Autodesk Inventor part; units mm, degrees
ref_plane "YZ Plane" through (0, 0, 0) normal (1, 0, 0) x (0, 1, 0)
ref_plane "XZ Plane" through (0, 0, 0) normal (0, 1, 0) x (-1, 0, 0)
ref_plane "XY Plane" through (0, 0, 0) normal (0, 0, 1) x (1, 0, 0)
sketch "スケッチ1" plane through (0, 0, 0) normal (0, 1, 0) x (-1, 0, 0)
  circle A0 centre (0, 0) radius 1.15
  circle A1 centre (0, 0) radius 1
  circle A2 centre (0, 0) radius 1.5
  circle A3 centre (0, 0) radius 2
  line L0 (1.5, 0) -> (1, 0)
  line L1 (1, 0) -> (1, 2)
  line L2 (1, 2) -> (1.5, 2)
  line L3 (1.5, 2) -> (1.5, 0)
  line L4 (0, 0) -> (5, 0)
  line L5 (5, 0) -> (5, -5)
  line L6 (5, -5) -> (0, -5)
  line L7 (0, -5) -> (0, 0)
  line L8 (5, -5) -> (0, -5)
  line L9 (0, -5) -> (0, 5)
  line L10 (0, 5) -> (5, 5)
  line L11 (5, 5) -> (5, -5)
  line L12 (0, 0) -> (-2, 0)
  line L13 (-2, 0) -> (-2, -5)
  line L14 (-2, -5) -> (0, -5)
  line L15 (0, -5) -> (0, 0)
  line L16 (-2, -5) -> (1.5, -5)
  line L17 (1.5, -5) -> (1.5, -1.5)
  line L18 (1.5, -1.5) -> (-2, -1.5)
  line L19 (-2, -1.5) -> (-2, -5)
  line L20 (1.5, 2) -> (-2, 2)
  line L21 (-2, 2) -> (-2, 5)
  line L22 (-2, 5) -> (1.5, 5)
  line L23 (1.5, 5) -> (1.5, 2)
  line L24 (-2, 2) -> (1.5, 2)
  line L25 (1.5, 2) -> (1.5, -1.5)
  line L26 (1.5, -1.5) -> (-2, -1.5)
  line L27 (-2, -1.5) -> (-2, 2)
  line L28 (0, -1) -> (-2, -1)
  line L29 (1.5, 2) -> (1, 2)
  line L30 (1, 2) -> (1, 5)
  line L31 (1, 5) -> (1.5, 5)
  line L32 (1.5, 5) -> (1.5, 2)
  line L33 (5, 5) -> (7, 5)
  line L34 (7, 5) -> (7, -5)
  line L35 (7, -5) -> (5, -5)
  line L36 (5, -5) -> (5, 5)
  line L37 (1, 0) -> (2, 0)
  line L38 (2, 0) -> (2, 5.3047)
  line L39 (2, 5.3047) -> (1, 5.3047)
  line L40 (1, 5.3047) -> (1, 0)
  line L41 (0, -2) -> (-2, -2)
  line L42 (-2, -2) -> (-2, -1)
  line L43 (-2, -1) -> (0, -1)
  line L44 (0, -1) -> (0, -2)
  point P0 (0, -1.5)
  point P1 (-2, -1.5)
  point P2 (0, 2)
  point P3 (1, 1.118)
  point P4 (-1.118, -1)
  point P5 (1.5, 5)
  point P6 (1, 1.7321)
  point P7 (-1.7321, -1)
  point P8 (2, 5)
  dimension "d2" = 3
  dimension "d3" = 4
  dimension "d0" = 2.3
  dimension "d1" = 2
  dimension "d4" = 5
  dimension "d5" = 5
  dimension "d6" = 10
  dimension "d15" = 2
extrude "押し出し1" add sketch "スケッチ1" along normal blind 5 contours L4 L5 L6 L17 L25 A3 | L38 L10 L11 L4 | L25 L18 A3 | A3 L20 L1 | A3 L18 L17 L6 L7 | L7 L14 L13 L41 | L11 L33 L34 L35 L5 | L20 L21 L22 L9 | L9 L10 L30 L20 | A3 L27 L20 | L28 L13 A3
extrude "押し出し2" add sketch "スケッチ1" along normal blind 0.6 contours L0 L1 A0 | L0 A2 L7 A0 | A0 L1 A2 L0 | A0 L7 A1 L0 | L1 A1 L9 A0 | A0 L9 A2 L1 | L7 A2 L28 A0 | A0 L28 L7 | L25 A3 L18 A2 | A2 L1 A3 L3 | L3 A3 L4 | L4 A3 L25 | L9 A1 L12 A0 | A0 L12 A2 L9 | A2 L9 A3 L1 | L28 A2 L12 A0 | A0 L12 A1 L28 | L18 A3 L28 A2 | L18 A3 L7 | L7 A3 L18 | L3 L23 L10 L38 A3 | A3 L1 L2 L3 | A2 L12 A3 L9 | L28 A3 L12 A2 | L41 L13 L18 A3 | L18 L13 L28 A3 | L2 L30 L10 L23
extrude "押し出し4" add sketch "スケッチ1" along normal blind 3.4 contours L41 L13 L18 A3 | L18 L13 L28 A3
sketch "スケッチ4" plane through (-7, 0, 5) normal (0, 0, 1) x (1, 0, 0)
  line L0 (9, 5) -> (0, 5)
  line L1 (0, 5) -> (2.5, 5)
  line L2 (2.5, 5) -> (2.5, 2.5)
  line L3 (2.5, 2.5) -> (0, 2.5)
  line L4 (0, 2.5) -> (0, 5)
  point P0 (7, 0)
  dimension "d25" = 2.5
  dimension "d26" = 2.5
hole "穴2" at (-4.5, 2.5, 5) direction (0, 0, -1) diameter 3.1 depth 8
properties part number "rod4.3"
Part model, mm, in its own coordinate system. A direction names the side the tool comes from. Coordinates: 2 decimals unless noted, no trailing zeros. Loops run counter-clockwise (first coordinate to the right, second up) from the corner with the lowest first, then second, coordinate; pieces in that order, holes last. Notation, with made-up numbers: (25, -18) -> (29, -18) arc R25 cw to (29, 17) -> close; hole circle Ø11 at (-32, 86.25). An arc over 180 degrees is marked (long way). Use a Markdown table: item, result. Add a question column.
Item 1: Band-saw the part on C-C on x = -4.5. Write the cut outline in (y, z).
Item 2: Band-saw the part on B-B on z = 0.75. Write the cut outline in (x, y).
Item 3: Flat gauge pins, fed straight in: P1, Ø4, axis at x = -0.5, z = -1, coming from the -Y side; P2, Ø3, axis at x = 0, z = 0, coming from the +Y side. Where does each tip first touch, or does it go through?
Item 4: Probe probe 1 along Y at (x, z) = (-4.5, -1); probe 2 along X at (y, z) = (3.1, 1); probe 3 along X at (y, z) = (1.8, 3). List the from-to ranges inside material, lowest first.
Item 5: Which spindle directions (+Z, -Z, +X, -X, +Y, -Y) get a long thin tool onto all of the face, cutting with end or side? Do faces 4 (the flat face through (-2, 3, 2)), 5 (the flat face through (-5, 3, -3)), 6 (the cylindrical face through (1.025, 2.769, 1.717)), 7 (the flat face through (1, 4, -2)). Say none if no direction does.
Item 6: Pull direction Y, two halves, no side cores. Call faces 1 (the flat face through (-2, 0, 0)), 2 (the cylindrical face through (-3.56, 3.73, 0.94)), 3 (the flat face through (-7, 2, 0)): +Y half, -Y half, draft (parallel to the pull), parting line (faces both ways), or undercut.
Item 7: Band-saw the part on D-D on x = 0.5. Write the cut outline in (y, z).
Geometry says:
| question | item | result |
|---|---|---|
| 1 | outline | (0, -5) -> (5, -5) -> (5, 5) -> (4.05, 5) -> (4.05, -3) -> (0.95, -3) -> (0.95, 5) -> (0, 5) -> close |
| 2 | outline | (-7, 0) -> (-0.66, 0) -> (-0.66, 0.6) -> (-2, 0.6) -> (-2, 5) -> (-7, 5) -> close; (0.66, 0) -> (2, 0) -> (2, 5) -> (1.85, 5) -> (1.85, 0.6) -> (0.66, 0.6) -> close; hole circle Ø3.1 at (-4.5, 2.5) |
| 3 | P1 | y = 0 |
| 3 | P2 | y = 0.6 |
| 4 | probe 1 | 0 to 0.95, 4.05 to 5 |
| 4 | probe 2 | -7 to -5.93, -3.07 to -2, 1.73 to 2 |
| 4 | probe 3 | -7 to -5.88, -3.12 to -2, -1 to 2 |
| 5 | face 4 | +Z, +Y |
| 5 | face 5 | +Z |
| 5 | face 6 | +Y |
| 5 | face 7 | +X, +Y |
| 6 | face 1 | -Y half |
| 6 | face 2 | undercut |
| 6 | face 3 | draft |
| 7 | outline | (0, -5) -> (5, -5) -> (5, -2) -> (3.4, -2) -> (3.4, -1.94) -> (0.6, -1.94) -> (0.6, -0.87) -> (0, -0.87) -> close; (0, 0.87) -> (0.6, 0.87) -> (0.6, 1.94) -> (5, 1.94) -> (5, 5) -> (0, 5) -> close |
